Input: part model. Units: mm. Frame: model coordinates. Face numbers are marked on the shaded views. A direction names the side the tool comes from. Coordinates: 2 decimals unless noted, no trailing zeros. Write each loop counter-clockwise with the first axis right and the second up, starting at its lowest first coordinate (ties: lowest second). Pieces come first, ordered by that corner, then holes.
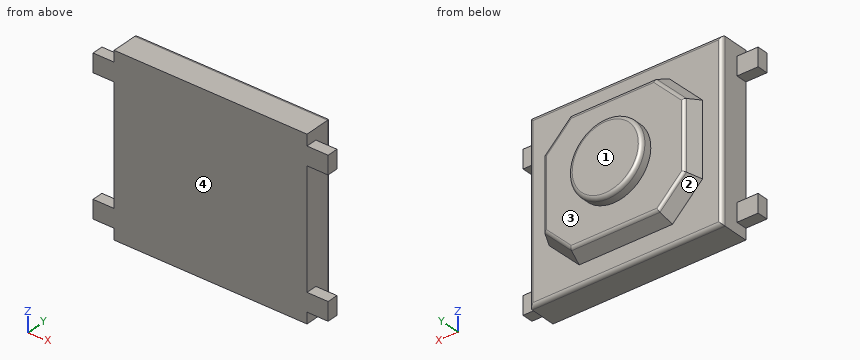
from build123d import *

# Parameters (mm, degrees)
SKETCH1_W               = 5.25
SKETCH1_H               = 4.8
BOSS_EXTRUDE1_DEPTH     = 0.8
BOSS_EXTRUDE2_DEPTH     = 0.4
SKETCH3_R               = 1
BOSS_EXTRUDE3_DEPTH     = 0.3
SKETCH4_W               = 0.5
SKETCH4_H               = 0.3
BOSS_EXTRUDE4_DEPTH     = 0.575
MIRROR2_COPY_1_SKETCH_W = 0.5
MIRROR2_COPY_1_SKETCH_H = 0.3
MIRROR2_COPY_1_DEPTH    = 0.575
DRAFT3_ANGLE            = 25
FILLET1_R               = 0.1
FILLET2_R               = 0.1


with BuildPart() as part:
    # Sketch1 → Boss-Extrude1 (new body)
    with BuildSketch(Plane(origin=(0, 0, 0), x_dir=(1, 0, 0), z_dir=(0, 1, 0))):
        Rectangle(SKETCH1_W, SKETCH1_H)
    extrude(amount=BOSS_EXTRUDE1_DEPTH)

    # Sketch2 → Boss-Extrude2 (add)
    with BuildSketch(Plane(origin=(0, 0.8, 0), x_dir=(1, 0, 0), z_dir=(0, 1, 0))):
        Polygon((-1.107585867, -1.67), (1.189705704, -1.67), (1.9, -0.959705704), (1.9, 0.962893219), (1.192893219, 1.67), (-1.192893219, 1.67), (-1.9, 0.962893219), (-1.9, -0.877585867), align=None)
    extrude(amount=BOSS_EXTRUDE2_DEPTH)

    # Sketch3 → Boss-Extrude3 (add)
    with BuildSketch(Plane(origin=(0, 1.2, 0), x_dir=(1, 0, 0), z_dir=(0, 1, 0))):
        with Locations(Location((0, 0, 0), (0, 0, 90))):
            Circle(SKETCH3_R)
    extrude(amount=BOSS_EXTRUDE3_DEPTH)

    # Sketch4 → Boss-Extrude4 (add)
    with BuildSketch(Plane(origin=(2.625, 0, 0), x_dir=(0, 0, -1), z_dir=(1, 0, 0))):
        with Locations((-1.85, 0.15)):
            Rectangle(SKETCH4_W, SKETCH4_H)
    boss_extrude4 = extrude(amount=BOSS_EXTRUDE4_DEPTH)

    # Mirror1: Boss-Extrude4 across plane
    add(boss_extrude4.mirror(Plane.XY))

    # Mirror2: Boss-Extrude4 across plane
    add(boss_extrude4.mirror(Plane(origin=(0, 0, 0), x_dir=(0, 0, 1), z_dir=(1, 0, 0))))

    # Mirror2 copy 1 sketch → Mirror2 copy 1 (add)
    with BuildSketch(Plane.ZY.offset(2.625)):
        with Locations((-1.85, 0.15)):
            Rectangle(MIRROR2_COPY_1_SKETCH_W, MIRROR2_COPY_1_SKETCH_H)
    extrude(amount=MIRROR2_COPY_1_DEPTH)

    # Draft3
    draft3_faces = [part.faces().sort_by_distance(p)[0] for p in [
        (1.544852852, 1, 1.314852852),
        (0.041059918, 1, 1.67),
        (-1.503792933, 1, 1.273792933),
        (-1.9, 1, -0.042653676),
        (-1.546446609, 1, -1.316446609),
        (0, 1, -1.67),
        (1.546446609, 1, -1.316446609),
        (1.9, 1, -0.001593757),
    ]]
    draft(draft3_faces, Plane(origin=(2.861299461, 1.2, -0.001593757), x_dir=(0, 0, 1), z_dir=(0, 1, 0)), DRAFT3_ANGLE)

    # Fillet1
    fillet1_edges = [part.edges().sort_by_distance(p)[0] for p in [
        (2.625, 0.8, 0),
        (0, 0.8, -2.4),
        (1.544852852, 1.2, 1.314852852),
        (1.9, 1.2, -0.001593757),
        (1.546446609, 1.2, -1.316446609),
        (0, 1.2, -1.67),
        (-1.546446609, 1.2, -1.316446609),
        (-1.9, 1.2, -0.042653676),
        (-1.503792933, 1.2, 1.273792933),
        (0.041059918, 1.2, 1.67),
        (-2.625, 0.8, 0),
        (0, 0.8, 2.4),
    ]]
    fillet(fillet1_edges, radius=FILLET1_R)

    # Fillet2
    fillet2_edges = [part.edges().sort_by_distance(p)[0] for p in [
        (0, 1.5, 1),
    ]]
    fillet(fillet2_edges, radius=FILLET2_R)


solid = part.part
Item 1: Pull-direction query (X, two-part tool) for the marked faces 1 and 2; classes: released by +X, released by -X, zero draft, split by the parting line, or undercut.
Item 2: Section query B-B, the plane z = 0. Return loops of the section in (x, y) (3 decimals), then the cut area to 3 significant figures.
Item 3: Access query for the marked faces 3 and 4. Directions: +Z, -Z, +X, -X, +Y, -Y. A direction counts if a zero-diameter tool reaches every point of the face in a straight line with its end or side. Return the directions, or none.
Item 4: Material intervals for line 1 (Y direction, x = -0.5, z = -1.2); line 2 (X direction, y = 0.3, z = -1.4) (3 decimals); line 3 (Y direction, x = 2.5, z = -1.7), sorted ascending.
Item 5: Section query A-A, the plane x = 3. Return loops of the section in (y, z), then the cut area to 3 significant figures.
Item 6: Section query C-C, the plane y = 0.2. Return loops of the section in (x, z) (3 decimals), then the cut area to 4 significant figures.
Item 7: Section query D-D, the plane x = 0. Return loops of the section in (y, z).
The answers:
1. face 1: zero draft
1. face 2: released by -X
2. outline: (-2.625, 0) - (2.625, 0) - (2.625, 0.7) arc R0.1 ccw to (2.525, 0.8) - (2.087, 0.8) - (1.927, 1.142) arc R0.1 ccw to (1.836, 1.2) - (1, 1.2) - (1, 1.4) arc R0.1 ccw to (0.9, 1.5) - (-0.9, 1.5) arc R0.1 ccw to (-1, 1.4) - (-1, 1.2) - (-1.836, 1.2) arc R0.1 ccw to (-1.927, 1.142) - (-2.087, 0.8) - (-2.525, 0.8) arc R0.1 ccw to (-2.625, 0.7) - close
2. area: 6.38 mm2
3. face 3: +Y
3. face 4: +Z, -Z, +X, -X, -Y
4. line 1: y = 0 to 1.2
4. line 2: x = -2.625 to 2.625
4. line 3: y = 0 to 0.8
5. outline: (0, -2.1) - (0.3, -2.1) - (0.3, -1.6) - (0, -1.6) - close; (0, 1.6) - (0.3, 1.6) - (0.3, 2.1) - (0, 2.1) - close
5. area: 0.300 mm2
6. outline: (-3.2, -2.1) - (-2.625, -2.1) - (-2.625, -2.4) - (2.625, -2.4) - (2.625, -2.1) - (3.2, -2.1) - (3.2, -1.6) - (2.625, -1.6) - (2.625, 1.6) - (3.2, 1.6) - (3.2, 2.1) - (2.625, 2.1) - (2.625, 2.4) - (-2.625, 2.4) - (-2.625, 2.1) - (-3.2, 2.1) - (-3.2, 1.6) - (-2.625, 1.6) - (-2.625, -1.6) - (-3.2, -1.6) - close
6. area: 26.35 mm2
7. outline: (0, -2.4) - (0.7, -2.4) arc R0.1 ccw to (0.8, -2.3) - (0.8, -1.86) - (1.14, -1.7) arc R0.1 ccw to (1.2, -1.61) - (1.2, -1) - (1.4, -1) arc R0.1 ccw to (1.5, -0.9) - (1.5, 0.9) arc R0.1 ccw to (1.4, 1) - (1.2, 1) - (1.2, 1.61) arc R0.1 ccw to (1.14, 1.7) - (0.8, 1.86) - (0.8, 2.3) arc R0.1 ccw to (0.7, 2.4) - (0, 2.4) - close
